Geometry: final body of the model. Coordinates: model frame, mm. Face numbers are marked on the shaded views. A direction names the side the tool comes from. Give positions to 0.01 mm unless a question says otherwise; leave off trailing zeros. Write each loop counter-clockwise with the first axis right and the second up, starting at its lowest first coordinate (ties: lowest second). Pieces come first, ordered by that corner, then holes. Notation, with made-up numbers: M -14.75,60.5 L 35.25,60.5 A15 cw 35.25,84.5 Z; hole C -23.5,5 d5. An arc over 180 degrees is marked long. One line per question, with ' | ' between items.
Solid Edge part; units mm, degrees
sketch "Sketch1" plane through (0, 0, 0) normal (0, 0, 1) x (1, 0, 0)
  line L0 (58, 49) -> (0, 49)
  line L1 (0, 49) -> (0, 0)
  line L2 (0, 0) -> (58, 0)
  line L3 (58, 0) -> (58, 49)
extrude "Protrusion1" add sketch "Sketch1" along normal blind 4
sketch "Sketch2" plane through (29, 24.5, 4) normal (0, 0, 1) x (1, 0, 0)
  circle A0 centre (-29, 24.5) radius 10
  circle A1 centre (29, 24.5) radius 10
extrude "Cutout1" cut sketch "Sketch2" against normal through all
sketch "Sketch3" plane through (29, 24.5, 4) normal (0, 0, 1) x (1, 0, 0)
  line L0 (-20, 10.5) -> (-29, 10.5)
  line L1 (-29, 10.5) -> (-29, 14.5)
  line L2 (-29, 14.5) -> (-20, 14.5)
  line L3 (-20, 14.5) -> (-20, 10.5)
  line L4 (20, 10.5) -> (29, 10.5)
  line L5 (29, 10.5) -> (29, 14.5)
  line L6 (29, 14.5) -> (20, 14.5)
  line L7 (20, 14.5) -> (20, 10.5)
extrude "ExtrudedProtrusion_2" add sketch "Sketch3" along normal blind 20
sketch "Sketch4" plane through (29, 24.5, 4) normal (0, 0, 1) x (1, 0, 0)
  line L0 (19, 10.5) -> (29, 10.5)
  line L1 (29, 10.5) -> (29, 0.5)
  line L2 (29, 0.5) -> (29, -24.5)
  line L3 (29, -24.5) -> (9, -24.5)
  line L4 (9, -24.5) -> (9, 0.5)
  arc A0 (9, 0.5) -> (19, 10.5) centre (19, 0.5) cw
extrude "Cutout2" cut sketch "Sketch4" against normal through all
sketch "Sketch5" plane through (0, 0, 0) normal (0, 0, 1) x (1, 0, 0)
  line L0 (52, -8) -> (52, 0)
  line L1 (0, 0) -> (52, 0)
  line L2 (0, 4) -> (0, 0)
  line L3 (52, 4) -> (0, 4)
  line L4 (52, 4) -> (56, 4)
  line L5 (56, 4) -> (56, -3)
  line L6 (94, -3) -> (56, -3)
  line L7 (94, -8) -> (94, -3)
  line L8 (56, -8) -> (94, -8)
  line L9 (56, -8) -> (52, -8)
extrude "ExtrudedProtrusion_3" add sketch "Sketch5" along normal blind 23
sketch "Sketch6" plane through (4.5, 39, 13.5) normal (0, 1, 0) x (-1, 0, 0)
  circle A0 centre (-49, 6) radius 2.5
  circle A1 centre (-49, -5) radius 2.5
  circle A2 centre (0, 6) radius 2.5
  circle A3 centre (0, -5) radius 2.5
extrude "Cutout3" cut sketch "Sketch6" against normal up to next
sketch "Sketch7" plane through (28, 4, 11.5) normal (0, 1, 0) x (-1, 0, 0)
  circle A0 centre (9, 2.5) radius 2.1
extrude "Cutout4" cut sketch "Sketch7" against normal up to next
fillet "Round_1" radius 4 2 edges at (56, 4, 11.5) (52, -8, 11.5)
sketch "Sketch8" plane through (47, -2, 23) normal (0, 0, 1) x (-1, 0, 0)
  line L0 (-47, 1) -> (-21, 1)
  line L1 (-21, 1) -> (-21, 6)
  line L2 (-21, 6) -> (-47, 6)
  line L3 (-47, 6) -> (-47, 1)
extrude "ExtrudedProtrusion_4" add sketch "Sketch8" along normal blind 5
fillet "Round_2" radius 14 3 edges at (94, -5.5, 28) (94, -5.5, 0) (68, -5.5, 28)
sketch "Sketch9" plane through (72, -3, 11.5) normal (0, 1, 0) x (0, 0, -1)
  circle A0 centre (-2.5, -7.5) radius 11
extrude "Cutout5" cut sketch "Sketch9" against normal up to next
sketch "Sketch10" plane through (75, -3, 14) normal (0, 1, 0) x (-1, 0, 0)
  line L0 (-2.5, 10.4979) -> (-6.5, 10.4979)
  line L1 (-6.5, 10.4979) -> (-6.5, 11.5021)
  line L2 (-6.5, 11.5021) -> (-2.5, 11.5021)
  line L3 (-2.5, 11.5021) -> (-2.5, 10.4979)
extrude "Cutout6" cut sketch "Sketch10" against normal through all
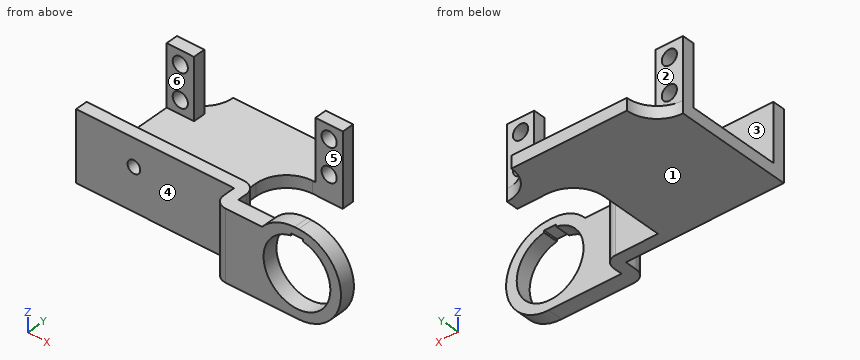
(1) Set-up query: the marked faces 4, 5 and 6. Return all of +Z, -Z, +X, -X, +Y, -Y with unobstructed straight access to the full face (end or side cutting, diameter ignored); none if empty.
Working result:
face 4: +Z, -Z, -X, -Y | face 5: +Z, -Z, +X | face 6: +Z, +X, -X
(2) Cut plane A-A, the plane x = 42. Return loops of the section in (y, z).
Working result:
outline: M 0,0 L 4,0 L 4,23 L 0,23 Z; M 33,0 L 49,0 L 49,4 L 33,4 Z
(3) Cut plane B-B, the plane z = 8.5. Count the separate pieces of the cut face and the enclosed holes in it, then the cut area to 3 significant figures.
Working result:
separate pieces: 6 | enclosed holes: 0 | area: 370 mm^2
(4) Cut plane D-D, the plane x = 19. Return loops of the section in (y, z).
Working result:
outline: M 0,0 L 49,0 L 49,4 L 4,4 L 4,11.9 L 0,11.9 Z; M 0,16.1 L 4,16.1 L 4,23 L 0,23 Z
(5) First-contact query: P1, Ø1.5, axis at x = 36.5, y = 23.5, coming from the +Z side; P2, Ø4.5, axis at y = 36.5, z = 15, coming from the +X side; P3, Ø4.5, axis at x = 4.5, z = 8.5, coming from the +Y side; P4, Ø3.5, axis at x = 41.5, y = -2, coming from the +Z side. Flat tips, straight axial feed; report the tip coordinate or a pass-through.
Working result:
P1: stops at z = 4 | P2: stops at x = 58 | P3: stops at y = 4 | P4: passes through
(6) Draft query along Y for the marked faces 1, 2 and 3. Return one class per face: released by +Y, released by -Y, zero draft, split by the parting line, or undercut.
Working result:
face 1: zero draft | face 2: released by +Y | face 3: undercut
(7) Cut plane C-C, the plane x = 53.5. Return loops of the section in (y, z).
Working result:
outline: M -7.12,0 L 3.71,0 L 3.71,23 L -7.12,23 Z; M 35,0 L 40.07,0 L 40.07,4 L 39,4 L 39,6 L 35,6 Z; M 35,11 L 39,11 L 39,17 L 35,17 Z; M 35,22 L 39,22 L 39,24 L 35,24 Z
(8) Material intervals for L1, parallel to Z at x = 4.5, y = 36.4; L2, parallel to Y at x = 50, z = 7; L3, parallel to Z at x = 19, y = 1.65, sorted ascending. Write a range as [from, to].
Working result:
L1: z = [0, 6], [11, 17], [22, 24] | L2: y = [0, 4], [35, 39] | L3: z = [0, 11.9], [16.1, 23]
